For this review, use the dimensioned drawing (mm, ordinates from the lowest corner) and the shaded views. Give positions to 0.01 mm unless a question says otherwise; leave off trailing zeros. Order: outer loops, then holes, each group sorted by start corner. A loop starts at its lowest first (then second) coordinate and runs counter-clockwise, first axis right, second up. Notation, with made-up numbers: (62.5, 44.5) - (120.5, 44.5) arc R15 ccw to (120.5, 65.5) - close; hole circle Ø10 at (57.25, 57.5). An arc over 180 degrees is marked (long way). Use a Markdown table: item, result. Add a question column.
1) We need section C-C on z = 42.5. Write out the cut boundary in (x, y), then the cut area to 3 significant figures.
2) We need section D-D on x = 2. Write out the cut boundary in (y, z), then the cut area to 3 significant figures.
3) We need section B-B on y = 23.5. Write out the cut boundary in (x, z), then the cut area to 3 significant figures.
4) Clearance check with flat-ended pins moving along their axes: P1, Ø1, axis at x = 11.5, z = 21.5, coming from the -Y side; P2, Ø6, axis at y = 12.5, z = 49, coming from the +X side; P3, Ø5, axis at y = 67.5, z = 34.5, coming from the +X side. State where each tip first meets the part, or that it passes through.
5) We need section A-A on x = 11.75. Write out the cut boundary in (y, z).
6) Wall thickness on L1, parallel to Z at x = 14.75, y = 12 (1 decimal); L2, parallel to Z at x = 21.5, y = 18.5; L3, parallel to X at y = 69.5, z = 27.5: over which ranges is each line inside the solid? List them lowest first.
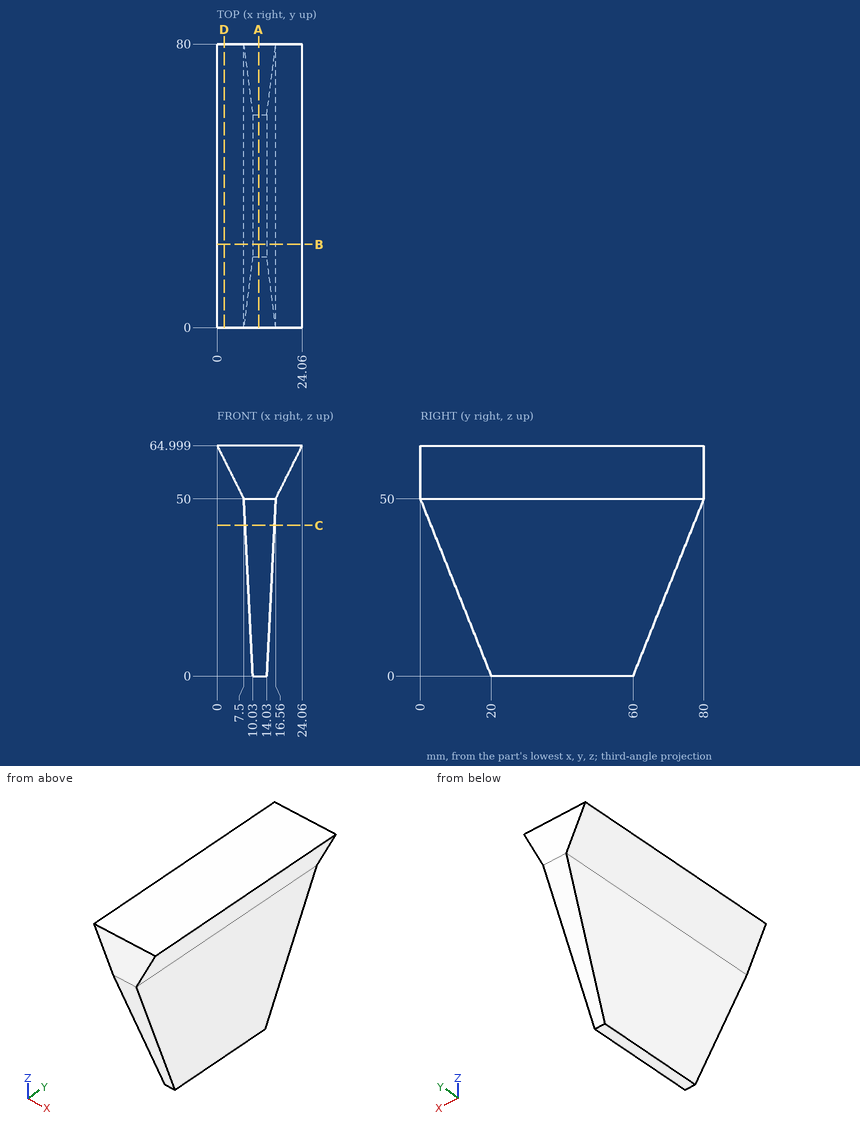
Checked values:
| question | item | result |
|---|---|---|
| 1 | outline | (7.88, 3) - (16.18, 3) - (16.18, 77) - (7.88, 77) - close |
| 1 | area | 614 mm² |
| 2 | outline | (0, 61) - (80, 61) - (80, 65) - (0, 65) - close |
| 2 | area | 320 mm² |
| 3 | outline | (0, 65) - (7.5, 50) - (10.03, 0) - (14.03, 0) - (16.56, 50) - (24.06, 65) - close |
| 3 | area | 575 mm² |
| 4 | P1 | y = 11.2 |
| 4 | P2 | x = 17.56 |
| 4 | P3 | x = 15.9 |
| 5 | outline | (0, 50) - (20, 0) - (60, 0) - (80, 50) - (80, 65) - (0, 65) - close |
| 6 | L1 | 20 to 65 |
| 6 | L2 | 59.88 to 65 |
| 6 | L3 | 8.64 to 15.42 |
